from build123d import *

# Parameters (mm, degrees)
BOSS_EXTRUDE1_DEPTH     = 100
CUT_EXTRUDE1_DEPTH      = 1968.929114577
CUT_EXTRUDE1_DEPTH_BACK = 1968.929114577
SKETCH3_W               = 33
SKETCH3_H               = 12
CAVITY1_START           = 619
CAVITY1_DEPTH           = 1


# Read off the part's stored shape, not the designer's step: Cavity1
with BuildPart() as part:
    # Sketch1 → Boss-Extrude1 (new body)
    with BuildSketch(Plane.XY):
        with BuildLine():
            Line((-13, 100), (-13, 1748))
            ThreePointArc((-13, 1748), (20.096933726, 1827.903066274), (100, 1861))
            Line((100, 1861), (519, 1861))
            ThreePointArc((519, 1861), (598.903066274, 1827.903066274), (632, 1748))
            Line((632, 1748), (632, 100))
            ThreePointArc((632, 100), (598.903066274, 20.096933726), (519, -13))
            Line((519, -13), (100, -13))
            ThreePointArc((100, -13), (20.096933726, 20.096933726), (-13, 100))
        make_face()
        with BuildLine():
            Line((100, 0), (519, 0))
            ThreePointArc((519, 0), (589.710678119, 29.289321881), (619, 100))
            Line((619, 100), (619, 1748))
            ThreePointArc((619, 1748), (589.710678119, 1818.710678119), (519, 1848))
            Line((519, 1848), (100, 1848))
            ThreePointArc((100, 1848), (29.289321881, 1818.710678119), (0, 1748))
            Line((0, 1748), (0, 100))
            ThreePointArc((0, 100), (29.289321881, 29.289321881), (100, 0))
        make_face(mode=Mode.SUBTRACT)
    extrude(amount=-BOSS_EXTRUDE1_DEPTH)

    # Sketch2 → Cut-Extrude1 (cut, two sides: drawn at the far end of the back side and taken through both)
    with BuildSketch(Plane(origin=(0, 0, 0), x_dir=(0, 0, -1), z_dir=(1, 0, 0)).offset(-CUT_EXTRUDE1_DEPTH_BACK)):
        with BuildLine():
            Line((100, 1861), (35, 1861))
            Line((35, 1861), (35, 123.590579564))
            ThreePointArc((35, 123.590579564), (51.869398873, 37.185139921), (100, -36.53))
            Line((100, -36.53), (100, 1861))
        make_face()
        with BuildLine():
            Line((0, -36.53), (53.916588263, -36.53))
            ThreePointArc((53.916588263, -36.53), (13.84098777, 39.113365936), (0, 123.590579564))
            Line((0, 123.590579564), (0, -36.53))
        make_face()
    extrude(amount=CUT_EXTRUDE1_DEPTH + CUT_EXTRUDE1_DEPTH_BACK, mode=Mode.SUBTRACT)

    # Cut-Sweep1: sweep along a curve in space
    with BuildLine() as cut_sweep1_path:
        ThreePointArc((-13, 123.590579564, -35), (-13, 111.779668745, -35.303826234), (-13, 100, -36.214501257))
        Line((-13, 1748, -35), (-13, 123.590579564, -35))
        ThreePointArc((100, 1861, -35), (20.096933726, 1827.903066274, -35), (-13, 1748, -35))
        Line((519, 1861, -35), (100, 1861, -35))
        ThreePointArc((632, 1748, -35), (598.903066274, 1827.903066274, -35), (519, 1861, -35))
        Line((632, 1748, -35), (632, 123.590579564, -35))
        ThreePointArc((632, 123.590579564, -35), (632, 111.779668745, -35.303826234), (632, 100, -36.214501257))
    # Sketch3 → Cut-Sweep1 (sweep, cut)
    with BuildSketch(Plane(origin=(309.5, 0, 0), x_dir=(0, 0, -1), z_dir=(1, 0, 0))):
        with Locations((17.5, 1855)):
            Rectangle(SKETCH3_W, SKETCH3_H)
    sweep(path=cut_sweep1_path.line, mode=Mode.SUBTRACT)

    # Cavity1 outline → Cavity1 (cut)
    with BuildSketch(Plane.YZ.offset(CAVITY1_START)):
        with BuildLine():
            ThreePointArc((1311, -33), (1311.707106781, -32.707106781), (1312, -32))
            Line((1312, -32), (1312, -26))
            ThreePointArc((1312, -26), (1311.707106781, -25.292893219), (1311, -25))
            Line((1311, -25), (1283, -25))
            ThreePointArc((1283, -25), (1282.292893219, -25.292893219), (1282, -26))
            Line((1282, -26), (1282, -32))
            ThreePointArc((1282, -32), (1282.292893219, -32.707106781), (1283, -33))
            Line((1283, -33), (1311, -33))
        make_face()
        with BuildLine():
            Line((501, -33), (529, -33))
            ThreePointArc((529, -33), (529.707106781, -32.707106781), (530, -32))
            Line((530, -32), (530, -26))
            ThreePointArc((530, -26), (529.707106781, -25.292893219), (529, -25))
            Line((529, -25), (501, -25))
            ThreePointArc((501, -25), (500.292893219, -25.292893219), (500, -26))
            Line((500, -26), (500, -32))
            ThreePointArc((500, -32), (500.292893219, -32.707106781), (501, -33))
        make_face()
    extrude(amount=CAVITY1_DEPTH, mode=Mode.SUBTRACT)


solid = part.part
Geometry: final body of the model. Coordinates: model frame, mm. A direction names the side the tool comes from. Round coordinates to 2 decimals unless told otherwise and drop trailing zeros. Loops run counter-clockwise (first coordinate to the right, second up) from the corner with the lowest first, then second, coordinate; pieces in that order, holes last. Notation, with made-up numbers: (36.5, 62.25) -> (88.5, 62.25) arc R8 cw to (88.5, 70.25) -> close; hole circle Ø5 at (43.25, 5). An arc over 180 degrees is marked (long way). One line per question, with ' | ' between items. Start each with the question number.
1. Section C-C on x = 34. Output: boundary loops of the cut face in (y, z), and give its area (3 significant figures).
2. Line query: line 1 along X through (y, z) = (1096, -6.5); line 2 along Y through (x, z) = (197, -39); line 3 along Y through (x, z) = (343, -17). Output: solid intervals per line, ascending. Write a range as [from, to].
3. Section B-B on y = 397. Output: boundary loops of the cut face in (x, z).
4. Mould query, pull axis Z, two halves, no side actions, for faces 5 (the face through (622, 996, 0)), 6 (the face through (312, 1848, -17)), 7 (the face through (-3, 996, -35)), 8 (the face through (622, 988, -34)). Classes: pulls with the +Z half, pulls with the -Z half, needs draft (parallel to the pull), parting line crosses it, or undercut.
5. Contact query for flat-ended pins moving along their axis: pin 1 (2 mm diameter, centred on x = 489, z = -64.5, fed in from +Y); pin 2 (1 mm diameter, centred on y = 1447, z = -17.5, fed in from +X); pin 3 (0.8 mm diameter, centred on x = 619.5, z = -29, fed in from -Y). Output: stop coordinate, or through.
6. Set-up query: faces 1 (the face through (590.484, 1817.929, -17.255)), 2 (the face through (-1, 911, -18)), 3 (the face through (599.777, 20.98, -39.984)), 4 (the face through (307, 1849, -17)). Return all of +Z, -Z, +X, -X, +Y, -Y with unobstructed straight access to the full face (end or side cutting, diameter ignored); none if empty.
7. Section A-A on x = 200. Output: boundary loops of the cut face in (y, z), and give its area (3 significant figures).
Returned:
1) outline: (8.28, -66.04) arc R229.72 cw to (24.87, -57.29) -> (24.87, -19.1) arc R264.72 ccw to (8.28, -26.44) -> close; (1823.13, -35) -> (1839.72, -35) -> (1839.72, -34) -> (1824.45, -34) -> (1824.45, -1) -> (1839.72, -1) -> (1839.72, 0) -> (1823.13, 0) -> close | area: 722 mm2
2) line 1: x = [-1, 0], [619, 620] | line 2: y = [-13, 0] | line 3: y = [1848, 1849]
3) outline: (-13, -35) -> (0, -35) -> (0, 0) -> (-13, 0) -> (-13, -1) -> (-1, -1) -> (-1, -34) -> (-13, -34) -> close; (619, -35) -> (632, -35) -> (632, -34) -> (620, -34) -> (620, -1) -> (632, -1) -> (632, 0) -> (619, 0) -> close
4) face 5: pulls with the +Z half | face 6: needs draft | face 7: pulls with the -Z half | face 8: undercut
5) pin 1: stops at y = 0 | pin 2: stops at x = 620 | pin 3: stops at y = 47.57
6) face 1: +Z, -Z | face 2: -X, +Y | face 3: +Z, -Z, +X, -Y | face 4: +X, -X, +Y
7) outline: (-13, -80.02) arc R229.72 cw to (0, -71.08) -> (0, -30.62) arc R264.72 ccw to (-13, -37.96) -> close; (1848, -35) -> (1861, -35) -> (1861, -34) -> (1849, -34) -> (1849, -1) -> (1861, -1) -> (1861, 0) -> (1848, 0) -> close | area: 595 mm2
